```python
from build123d import *

# Parameters (mm, degrees)
PLATFORM_W                   = 50
PLATFORM_H                   = 72
PLATFORM_W_2                 = 22.5
PLATFORM_H_2                 = 43
PLATFORM_HEIGHT_DEPTH        = 2
TUBE_OUTER_DIAMETER_SKETCH_R = 1.5
TUBE_START                   = -6.464466201
TUBE_INNER_DIAMETER_DEPTH    = 10.707106612
FILLET1_R                    = 2


# Read off the part's stored shape, not the designer's step: Tube Inner Diameter
with BuildPart() as part:
    # Platform → Platform Height (new body)
    # profile 1 of 2: a face of its own
    with BuildSketch(Plane(origin=(0, 0, 0), x_dir=(1, 0, 0), z_dir=(0, 1, 0))):
        Rectangle(PLATFORM_W, PLATFORM_H)
        Rectangle(PLATFORM_W_2, PLATFORM_H_2, mode=Mode.SUBTRACT)
    # profile 2 of 2: a face of its own
    with BuildSketch(Plane(origin=(0, 0, 0), x_dir=(1, 0, 0), z_dir=(0, 1, 0))):
        Rectangle(PLATFORM_W_2, PLATFORM_H_2)
    extrude(amount=PLATFORM_HEIGHT_DEPTH)

    # Tube Outer Diameter: sweep along a curve in space
    with BuildLine() as tube_outer_diameter_path:
        Line((0, 2, -3.5), (0, -5.071067812, 3.571067812))
    # Tube Outer Diameter Sketch → Tube Outer Diameter (sweep)
    with BuildSketch(Plane(origin=(0, 2, 0), x_dir=(1, 0, 0), z_dir=(0, 1, 0))):
        with Locations((0, 3.5)):
            Circle(TUBE_OUTER_DIAMETER_SKETCH_R)
    sweep(path=tube_outer_diameter_path.line)

    # Tube Inner Diameter outline → Tube Inner Diameter (cut)
    with BuildSketch(Plane(origin=(0, 0, 0), x_dir=(1, 0, 0), z_dir=(0, 0.7071067811865487, -0.7071067811865464)).offset(TUBE_START)):
        with BuildLine():
            add(Edge.make_bspline(
                [(0, 0.707106781), (1, 0.707106781), (1, 1.414213562), (0, 1.414213562), (-1, 1.414213562), (-1, 0.707106781), (0, 0.707106781)],
                knots=[0, 0, 0, 0, 0.5, 0.5, 0.5, 1, 1, 1, 1], degree=3, weights=[1, 0.333333333, 0.333333333, 1, 0.333333333, 0.333333333, 1]))
        make_face()
    extrude(amount=TUBE_INNER_DIAMETER_DEPTH, mode=Mode.SUBTRACT)

    # Fillet1
    fillet1_edges = [part.edges().sort_by_distance(p)[0] for p in [
        (-25, 1, 36),
        (-25, 1, -36),
        (25, 1, -36),
        (25, 1, 36),
    ]]
    fillet(fillet1_edges, radius=FILLET1_R)


solid = part.part
```
The listing builds one solid part. Answer for the finished solid, in the listing's coordinates (mm). Give positions to 0.01 mm unless a question says otherwise; leave off trailing zeros. Order: outer loops, then holes, each group sorted by start corner. A loop starts at its lowest first (then second) coordinate and runs counter-clockwise, first axis right, second up. Notation, with made-up numbers: (86, 14) - (138, 14) arc R15 cw to (138, 30) - close; hole circle Ø9 at (-19, 3). An arc over 180 degrees is marked (long way). Answer in a Markdown table with one row per item. Add a question column.
Q1. For a pull along Z with two mould halves and no side action, classify faces 1 (the flat face through (25, 1, 0)), 2 (the cylindrical face through (-24.4, 1.01, -35.43)), 3 (the flat face through (0, 1, 36)) as released by +Z, released by -Z, zero draft, split by the parting line, or undercut.
Q2. The part is cut by section C-C (z = 11.5). Determine the outline of the cut face in (x, y).
Q3. The part is cut by section B-B (x = -14). Determine the outline of the cut face in (y, z), then the cut area to 3 significant figures.
Q4. The part is cut by section A-A (z = 1). Give the number of separate pieces and of enclosed holes in the cut face, then the cut area to 3 significant figures.
Q5. Given P1, Ø15, axis at x = -12, z = 14, coming from the -Y side, flat-ended and moving along its own axis, determine where the tip first touches the part or whether it passes through.
Q6. Find the intervals of material crossed by line 1 along Y through (x, z) = (-20, 24); line 2 along X through (y, z) = (-2, 1.5), in increasing order. Write a range as [from, to].
Determined:
| question | item | result |
|---|---|---|
| 1 | face 1 | zero draft |
| 1 | face 2 | released by -Z |
| 1 | face 3 | released by +Z |
| 2 | outline | (-25, 0) - (25, 0) - (25, 2) - (-25, 2) - close |
| 3 | outline | (0, -36) - (2, -36) - (2, 36) - (0, 36) - close |
| 3 | area | 144 mm² |
| 4 | separate pieces | 2 |
| 4 | enclosed holes | 1 |
| 4 | area | 106 mm² |
| 5 | P1 | stops at y = 0 |
| 6 | line 1 | y = [0, 2] |
| 6 | line 2 | x = [-1.12, 1.12] |
